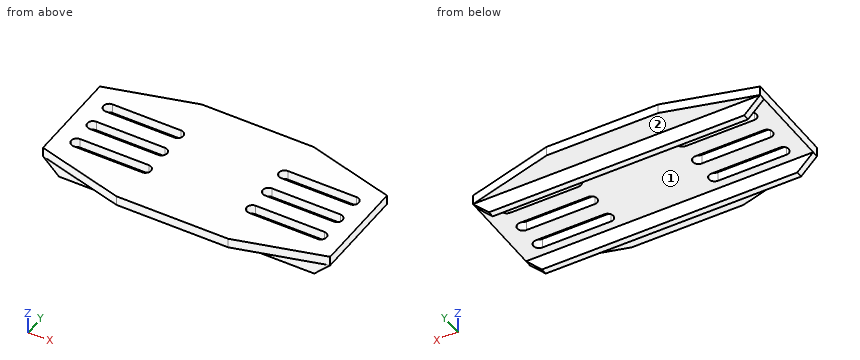
from build123d import *

# Parameters (mm, degrees)
F0_W     = 45
F0_H     = 2
F1_DEPTH = 3
F2_DEPTH = 5
F3_SIZE  = 5


with BuildPart() as f1:
    # F0 (on Top) → F1 (new body)
    with BuildSketch(Plane.XY):
        Polygon((-47.8720533848, 45), (-65.3720533848, 45), (-92.8720533848, 37.5), (-47.8720533848, 37.5), align=None)
        Polygon((-30.3720533848, 45), (-47.8720533848, 45), (-47.8720533848, 37.5), (-2.8720533848, 37.5), align=None)
        with Locations((-70.3720533848, 36.5)):
            Rectangle(F0_W, F0_H)
        with Locations((-25.3720533848, 36.5)):
            Rectangle(F0_W, F0_H)
        with BuildLine():
            Line((-47.8720533848, 35.5), (-92.8720533848, 35.5))
            Line((-92.8720533848, 35.5), (-92.8720533848, 31))
            Line((-92.8720533848, 31), (-87.8720533848, 31))
            ThreePointArc((-87.8720533848, 31), (-87.3594902519, 32.2374368671), (-86.1220533848, 32.75))
            Line((-86.1220533848, 32.75), (-64.6220533848, 32.75))
            ThreePointArc((-64.6220533848, 32.75), (-63.3846165177, 32.2374368671), (-62.8720533848, 31))
            Line((-62.8720533848, 31), (-47.8720533848, 31))
            Line((-47.8720533848, 31), (-47.8720533848, 35.5))
        make_face()
        with BuildLine():
            Line((-2.8720533848, 35.5), (-47.8720533848, 35.5))
            Line((-47.8720533848, 35.5), (-47.8720533848, 31))
            Line((-47.8720533848, 31), (-32.8720533848, 31))
            ThreePointArc((-32.8720533848, 31), (-32.3594902519, 32.2374368671), (-31.1220533848, 32.75))
            Line((-31.1220533848, 32.75), (-9.6220533848, 32.75))
            ThreePointArc((-9.6220533848, 32.75), (-8.3846165177, 32.2374368671), (-7.8720533848, 31))
            Line((-7.8720533848, 31), (-2.8720533848, 31))
            Line((-2.8720533848, 31), (-2.8720533848, 35.5))
        make_face()
        with BuildLine():
            Line((-87.8720533848, 31), (-92.8720533848, 31))
            Line((-92.8720533848, 31), (-92.8720533848, 22.5))
            Line((-92.8720533848, 22.5), (-87.8720533848, 22.5))
            ThreePointArc((-87.8720533848, 22.5), (-87.3594902519, 23.7374368671), (-86.1220533848, 24.25))
            Line((-86.1220533848, 24.25), (-64.6220533848, 24.25))
            ThreePointArc((-64.6220533848, 24.25), (-63.3846165177, 23.7374368671), (-62.8720533848, 22.5))
            Line((-62.8720533848, 22.5), (-47.8720533848, 22.5))
            Line((-47.8720533848, 22.5), (-47.8720533848, 31))
            Line((-47.8720533848, 31), (-62.8720533848, 31))
            ThreePointArc((-62.8720533848, 31), (-63.3846165177, 29.7625631329), (-64.6220533848, 29.25))
            Line((-64.6220533848, 29.25), (-86.1220533848, 29.25))
            ThreePointArc((-86.1220533848, 29.25), (-87.3594902519, 29.7625631329), (-87.8720533848, 31))
        make_face()
        with BuildLine():
            Line((-32.8720533848, 31), (-47.8720533848, 31))
            Line((-47.8720533848, 31), (-47.8720533848, 22.5))
            Line((-47.8720533848, 22.5), (-32.8720533848, 22.5))
            ThreePointArc((-32.8720533848, 22.5), (-32.3594902519, 23.7374368671), (-31.1220533848, 24.25))
            Line((-31.1220533848, 24.25), (-9.6220533848, 24.25))
            ThreePointArc((-9.6220533848, 24.25), (-8.3846165177, 23.7374368671), (-7.8720533848, 22.5))
            Line((-7.8720533848, 22.5), (-2.8720533848, 22.5))
            Line((-2.8720533848, 22.5), (-2.8720533848, 31))
            Line((-2.8720533848, 31), (-7.8720533848, 31))
            ThreePointArc((-7.8720533848, 31), (-8.3846165177, 29.7625631329), (-9.6220533848, 29.25))
            Line((-9.6220533848, 29.25), (-31.1220533848, 29.25))
            ThreePointArc((-31.1220533848, 29.25), (-32.3594902519, 29.7625631329), (-32.8720533848, 31))
        make_face()
        with BuildLine():
            Line((-87.8720533848, 22.5), (-92.8720533848, 22.5))
            Line((-92.8720533848, 22.5), (-92.8720533848, 14))
            Line((-92.8720533848, 14), (-87.8720533848, 14))
            ThreePointArc((-87.8720533848, 14), (-87.3594902519, 15.2374368671), (-86.1220533848, 15.75))
            Line((-86.1220533848, 15.75), (-64.6220533848, 15.75))
            ThreePointArc((-64.6220533848, 15.75), (-63.3846165177, 15.2374368671), (-62.8720533848, 14))
            Line((-62.8720533848, 14), (-47.8720533848, 14))
            Line((-47.8720533848, 14), (-47.8720533848, 22.5))
            Line((-47.8720533848, 22.5), (-62.8720533848, 22.5))
            ThreePointArc((-62.8720533848, 22.5), (-63.3846165177, 21.2625631329), (-64.6220533848, 20.75))
            Line((-64.6220533848, 20.75), (-86.1220533848, 20.75))
            ThreePointArc((-86.1220533848, 20.75), (-87.3594902519, 21.2625631329), (-87.8720533848, 22.5))
        make_face()
        with BuildLine():
            Line((-32.8720533848, 22.5), (-47.8720533848, 22.5))
            Line((-47.8720533848, 22.5), (-47.8720533848, 14))
            Line((-47.8720533848, 14), (-32.8720533848, 14))
            ThreePointArc((-32.8720533848, 14), (-32.3594902519, 15.2374368671), (-31.1220533848, 15.75))
            Line((-31.1220533848, 15.75), (-9.6220533848, 15.75))
            ThreePointArc((-9.6220533848, 15.75), (-8.3846165177, 15.2374368671), (-7.8720533848, 14))
            Line((-7.8720533848, 14), (-2.8720533848, 14))
            Line((-2.8720533848, 14), (-2.8720533848, 22.5))
            Line((-2.8720533848, 22.5), (-7.8720533848, 22.5))
            ThreePointArc((-7.8720533848, 22.5), (-8.3846165177, 21.2625631329), (-9.6220533848, 20.75))
            Line((-9.6220533848, 20.75), (-31.1220533848, 20.75))
            ThreePointArc((-31.1220533848, 20.75), (-32.3594902519, 21.2625631329), (-32.8720533848, 22.5))
        make_face()
        with BuildLine():
            Line((-87.8720533848, 14), (-92.8720533848, 14))
            Line((-92.8720533848, 14), (-92.8720533848, 9.5))
            Line((-92.8720533848, 9.5), (-47.8720533848, 9.5))
            Line((-47.8720533848, 9.5), (-47.8720533848, 14))
            Line((-47.8720533848, 14), (-62.8720533848, 14))
            ThreePointArc((-62.8720533848, 14), (-63.3846165177, 12.7625631329), (-64.6220533848, 12.25))
            Line((-64.6220533848, 12.25), (-86.1220533848, 12.25))
            ThreePointArc((-86.1220533848, 12.25), (-87.3594902519, 12.7625631329), (-87.8720533848, 14))
        make_face()
        with BuildLine():
            Line((-32.8720533848, 14), (-47.8720533848, 14))
            Line((-47.8720533848, 14), (-47.8720533848, 9.5))
            Line((-47.8720533848, 9.5), (-2.8720533848, 9.5))
            Line((-2.8720533848, 9.5), (-2.8720533848, 14))
            Line((-2.8720533848, 14), (-7.8720533848, 14))
            ThreePointArc((-7.8720533848, 14), (-8.3846165177, 12.7625631329), (-9.6220533848, 12.25))
            Line((-9.6220533848, 12.25), (-31.1220533848, 12.25))
            ThreePointArc((-31.1220533848, 12.25), (-32.3594902519, 12.7625631329), (-32.8720533848, 14))
        make_face()
        with Locations((-70.3720533848, 8.5)):
            Rectangle(F0_W, F0_H)
        with Locations((-25.3720533848, 8.5)):
            Rectangle(F0_W, F0_H)
        Polygon((-47.8720533848, 7.5), (-92.8720533848, 7.5), (-65.3720533848, 0), (-47.8720533848, 0), align=None)
        Polygon((-2.8720533848, 7.5), (-47.8720533848, 7.5), (-47.8720533848, 0), (-30.3720533848, 0), align=None)
    extrude(amount=F1_DEPTH)

    # F0 (on Top) → F2 (join)
    with BuildSketch(Plane.XY):
        with Locations((-25.3720533848, 36.5)):
            Rectangle(F0_W, F0_H)
        with Locations((-70.3720533848, 36.5)):
            Rectangle(F0_W, F0_H)
        with Locations((-25.3720533848, 8.5)):
            Rectangle(F0_W, F0_H)
        with Locations((-70.3720533848, 8.5)):
            Rectangle(F0_W, F0_H)
    extrude(amount=-F2_DEPTH)

    # F3
    f3_edges = [f1.edges().sort_by_distance(p)[0] for p in [
        (-92.872053, 36.5, -5),
        (-92.872053, 8.5, -5),
        (-2.872053, 8.5, -5),
        (-2.872053, 36.5, -5),
    ]]
    chamfer(f3_edges, length=F3_SIZE)


solid = f1.part
Verification items for the finished model (mm, model axes). Face numbers are marked on the shaded views. Give positions to 0.01 mm unless a question says otherwise; leave off trailing zeros. Write each loop counter-clockwise with the first axis right and the second up, starting at its lowest first coordinate (ties: lowest second). Pieces come first, ordered by that corner, then holes. Notation, with made-up numbers: M 36,89.25 L 71,89.25 A16 cw 71,104.25 Z; hole C 38.25,33 d4. An arc over 180 degrees is marked long. Write item = value, one per line.
(1) Sectioned sample at B-B (x = -28). Record the cut outline in (y, z).
Found:
outline = M 0.65,0 L 7.5,0 L 7.5,-5 L 9.5,-5 L 9.5,0 L 12.25,0 L 12.25,3 L 0.65,3 Z; M 15.75,0 L 20.75,0 L 20.75,3 L 15.75,3 Z; M 24.25,0 L 29.25,0 L 29.25,3 L 24.25,3 Z; M 32.75,0 L 35.5,0 L 35.5,-5 L 37.5,-5 L 37.5,0 L 44.35,0 L 44.35,3 L 32.75,3 Z
(2) Draft check along Y on the marked faces 1 and 2. Enter one of: released by +Y, released by -Y, zero draft, split by the parting line, or undercut.
Found:
face_1 = undercut
face_2 = zero draft
(3) Sectioned sample at C-C (x = -53). Record the cut outline in (y, z).
Found:
outline = M 0,0 L 7.5,0 L 7.5,-5 L 9.5,-5 L 9.5,0 L 35.5,0 L 35.5,-5 L 37.5,-5 L 37.5,0 L 45,0 L 45,3 L 0,3 Z
(4) Sectioned sample at D-D (y = 18). Record the cut outline in (x, z), then the cut area to 3 significant figures.
Found:
outline = M -92.87,0 L -2.87,0 L -2.87,3 L -92.87,3 Z
area = 270 mm2
(5) Material ranges on line 1 (Y direction, x = -35.5, z = -4.5); line 2 (Y direction, x = -80, z = 2.25); line 3 (Z direction, x = -35, y = 16), recorded low to high.
Found:
line_1 = 7.5 to 9.5, 35.5 to 37.5
line_2 = 3.99 to 12.25, 15.75 to 20.75, 24.25 to 29.25, 32.75 to 41.01
line_3 = 0 to 3
(6) Sectioned sample at A-A (z = -2.5). Record the cut outline in (x, y), then the cut area to 3 significant figures.
Found:
outline = M -90.37,7.5 L -5.37,7.5 L -5.37,9.5 L -90.37,9.5 Z; M -90.37,35.5 L -5.37,35.5 L -5.37,37.5 L -90.37,37.5 Z
area = 340 mm2
(7) Go/stop test with flat-tipped pins: pin 1 Ø3.5 at (x, z) = (-72, 1.5) entering from -Y; pin 2 Ø2.5 at (x, z) = (-16, 1) entering from +Y; pin 3 Ø1.5 at (x, z) = (-48, -2.5) entering from +Y. Record where each tip stops, or that it passes through.
Found:
pin_1 = 1.33
pin_2 = 41.42
pin_3 = 37.5
